Part model, mm, in its own coordinate system. A direction names the side the tool comes from. Coordinates: 2 decimals unless noted, no trailing zeros. Write each loop counter-clockwise with the first axis right and the second up, starting at its lowest first coordinate (ties: lowest second). Pieces come first, ordered by that corner, then holes. Notation, with made-up numbers: (83.25, 40.25) - (101.25, 40.25) arc R22 cw to (101.25, 62.25) - close; hole circle Ø4 at (-34.5, 86). An arc over 180 degrees is marked (long way). Use a Markdown table: item, result.
```python
from build123d import *

# Parameters (mm, degrees)
SKETCH3_W          = 114
SKETCH3_H          = 95
EXTRUDE1_DEPTH     = 1.6
SKETCH4_W          = 7.4
SKETCH4_H          = 36.6
EXTRUDE2_DEPTH     = 9.5
SKETCH5_R          = 1.35
EXTRUDE3_DEPTH     = 7
SKETCH7_W          = 114
SKETCH7_H          = 95
EXTRUDE4_DEPTH     = 1
SKETCH8_R          = 1
CUT_EXTRUDE1_DEPTH = 20.1


with BuildPart() as part:
    # Sketch3 → Extrude1 (new body)
    with BuildSketch(Plane(origin=(0, 0, 0), x_dir=(1, 0, 0), z_dir=(0, 1, 0))):
        Rectangle(SKETCH3_W, SKETCH3_H)
    extrude(amount=EXTRUDE1_DEPTH)

    # Sketch4 → Extrude2 (add)
    with BuildSketch(Plane.XZ):
        with Locations((-52.8, 21.7)):
            Rectangle(SKETCH4_W, SKETCH4_H)
        with Locations((-52.8, -24.1)):
            Rectangle(SKETCH4_W, SKETCH4_H)
        with Locations((52.8, 21.7)):
            Rectangle(SKETCH4_W, SKETCH4_H)
        with Locations((52.8, -19.9)):
            Rectangle(SKETCH4_W, SKETCH4_H)
    extrude(amount=EXTRUDE2_DEPTH)

    # Sketch5 → Extrude3 (add)
    with BuildSketch(Plane(origin=(0, 1.6, 0), x_dir=(-1, 0, 0), z_dir=(0, 1, 0))):
        with Locations((54, -45)):
            Circle(SKETCH5_R)
        with Locations((54, 45)):
            Circle(SKETCH5_R)
        with Locations((-54, 45)):
            Circle(SKETCH5_R)
        with Locations((-54, -45)):
            Circle(SKETCH5_R)
    extrude(amount=EXTRUDE3_DEPTH)

    # Sketch7 → Extrude4 (add)
    with BuildSketch(Plane(origin=(0, 8.6, 0), x_dir=(-1, 0, 0), z_dir=(0, 1, 0))):
        Rectangle(SKETCH7_W, SKETCH7_H)
    extrude(amount=EXTRUDE4_DEPTH)

    # Sketch8 → Cut-Extrude1 (cut, through all)
    with BuildSketch(Plane(origin=(0, 9.6, 0), x_dir=(-1, 0, 0), z_dir=(0, 1, 0))):
        with Locations((54, -45)):
            Circle(SKETCH8_R)
        with Locations((54, 45)):
            Circle(SKETCH8_R)
        with Locations((-54, 45)):
            Circle(SKETCH8_R)
        with Locations((-54, -45)):
            Circle(SKETCH8_R)
    extrude(amount=-CUT_EXTRUDE1_DEPTH, mode=Mode.SUBTRACT)


solid = part.part
```
Item 1: Band-saw the part on A-A, the plane y = 6. Give the cut face in (x, z).
From the geometry:
| item | result |
|---|---|
| outline | circle Ø2.7 at (-54, -45); circle Ø2.7 at (-54, 45); circle Ø2.7 at (54, -45); circle Ø2.7 at (54, 45); hole circle Ø2 at (-54, -45); hole circle Ø2 at (-54, 45); hole circle Ø2 at (54, -45); hole circle Ø2 at (54, 45) |
Item 2: Two-plate mould, pull along X, no slides. Class faces 1 (the face through (-53.71, 5.05, -46.32)), 2 (the face through (-53, -5, 40)), 3 (the face through (56.5, -5, 21)): pulls with the +X half, pulls with the -X half, needs draft (parallel to the pull), parting line crosses it, or undercut.
From the geometry:
| item | result |
|---|---|
| face 1 | undercut |
| face 2 | needs draft |
| face 3 | pulls with the +X half |
Item 3: Band-saw the part on C-C, the plane z = -21.5. Give the cut face in (x, y), then the cut area to 3 significant figures.
From the geometry:
| item | result |
|---|---|
| outline | (-57, 0) - (-56.5, 0) - (-56.5, -9.5) - (-49.1, -9.5) - (-49.1, 0) - (49.1, 0) - (49.1, -9.5) - (56.5, -9.5) - (56.5, 0) - (57, 0) - (57, 1.6) - (-57, 1.6) - close; (-57, 8.6) - (57, 8.6) - (57, 9.6) - (-57, 9.6) - close |
| area | 437 mm^2 |
Item 4: Band-saw the part on D-D, the plane y = -7.5. Give the cut face in (x, z), then the cut area to 3 significant figures.
From the geometry:
| item | result |
|---|---|
| outline | (-56.5, -42.4) - (-49.1, -42.4) - (-49.1, -5.8) - (-56.5, -5.8) - close; (-56.5, 3.4) - (-49.1, 3.4) - (-49.1, 40) - (-56.5, 40) - close; (49.1, -38.2) - (56.5, -38.2) - (56.5, -1.6) - (49.1, -1.6) - close; (49.1, 3.4) - (56.5, 3.4) - (56.5, 40) - (49.1, 40) - close |
| area | 1,080 mm^2 |
Item 5: Band-saw the part on B-B, the plane x = 39.5. Give the cut face in (y, z), then the cut area to 3 significant figures.
From the geometry:
| item | result |
|---|---|
| outline | (0, -47.5) - (1.6, -47.5) - (1.6, 47.5) - (0, 47.5) - close; (8.6, -47.5) - (9.6, -47.5) - (9.6, 47.5) - (8.6, 47.5) - close |
| area | 247 mm^2 |
Item 6: Drop flat-ended pins along their axis: P1, Ø2.5, axis at x = -54, z = -45, coming from the +Y side; P2, Ø2, axis at y = -3.5, z = 7, coming from the -X side; P3, Ø3.5, axis at x = -54, y = -5.5, coming from the -Z side; P4, Ø6, axis at x = -54.5, y = -3.5, coming from the +Z side. Give the stop position or say it passes through.
From the geometry:
| item | result |
|---|---|
| P1 | y = 9.6 |
| P2 | x = -56.5 |
| P3 | z = -42.4 |
| P4 | z = 40 |
Item 7: Which spindle directions (+Z, -Z, +X, -X, +Y, -Y) get a long thin tool onto all of the face, cutting with end or side? Do faces 4 (the face through (-53, -5, -42.4)), 5 (the face through (-49.1, -5, 21)), 6 (the face through (54.29, 5.05, 43.68)). Say none if no direction does.
From the geometry:
| item | result |
|---|---|
| face 4 | -Z, +X, -X, -Y |
| face 5 | +Z, -Z, -Y |
| face 6 | none |
Item 8: Drill centre lines: probe 1 along Z at (x, y) = (-54, 5.25); probe 2 along Y at (x, z) = (16, 16); probe 3 along Z at (x, y) = (51.5, -3.75). Where is each one in solid material? Low to high.
From the geometry:
| item | result |
|---|---|
| probe 1 | -46.35 to -46, -44 to -43.65, 43.65 to 44, 46 to 46.35 |
| probe 2 | 0 to 1.6, 8.6 to 9.6 |
| probe 3 | -38.2 to -1.6, 3.4 to 40 |
